Here's the drawing with two shaded views (mm, measured from the low corner). I have some questions. A direction names the side the tool comes from. Coordinates: 2 decimals unless noted, no trailing zeros. Loops run counter-clockwise (first coordinate to the right, second up) from the corner with the lowest first, then second, coordinate; pieces in that order, holes last. Notation, with made-up numbers: (11, -0.75) - (60, -0.75) arc R23 ccw to (60, 16.25) - close; hole circle Ø9 at (56.25, -13). An arc over 180 degrees is marked (long way). Use a Markdown table: item, result.
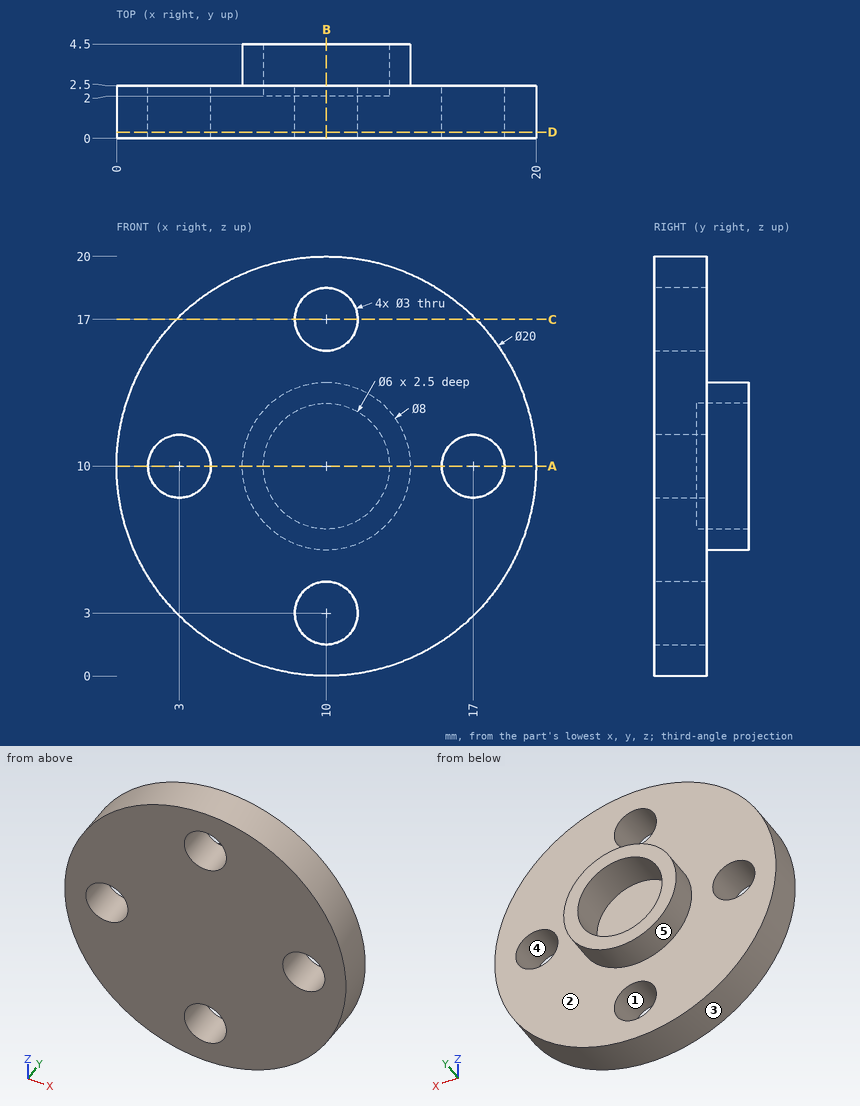
Q1. Will these pins go through, and if not, where does the flat tip stop? P1, Ø2, axis at x = 4, z = 3, coming from the +Y side; P2, Ø3, axis at x = 10, z = 9.5, coming from the +Y side.
Check values:
| item | result |
|---|---|
| P1 | y = 2.5 |
| P2 | y = 2 |
Q2. I want a section at D-D, the plane y = 0.3. Write out the boundary of the cut face in (x, z).
Check values:
| item | result |
|---|---|
| outline | circle Ø20 at (10, 10); hole circle Ø3 at (3, 10); hole circle Ø3 at (10, 3); hole circle Ø3 at (10, 17); hole circle Ø3 at (17, 10) |
Q3. I want a section at B-B, the plane x = 10. Write out the boundary of the cut face in (y, z).
Check values:
| item | result |
|---|---|
| outline | (0, 0) - (2.5, 0) - (2.5, 1.5) - (0, 1.5) - close; (0, 4.5) - (2.5, 4.5) - (2.5, 6) - (4.5, 6) - (4.5, 7) - (2, 7) - (2, 13) - (4.5, 13) - (4.5, 14) - (2.5, 14) - (2.5, 15.5) - (0, 15.5) - close; (0, 18.5) - (2.5, 18.5) - (2.5, 20) - (0, 20) - close |
Q4. I want a section at C-C, the plane z = 17. Write out the boundary of the cut face in (x, y).
Check values:
| item | result |
|---|---|
| outline | (2.86, 0) - (8.5, 0) - (8.5, 2.5) - (2.86, 2.5) - close; (11.5, 0) - (17.14, 0) - (17.14, 2.5) - (11.5, 2.5) - close |
Q5. I want a section at A-A, the plane z = 10. Write out the boundary of the cut face in (x, y).
Check values:
| item | result |
|---|---|
| outline | (0, 0) - (1.5, 0) - (1.5, 2.5) - (0, 2.5) - close; (4.5, 0) - (15.5, 0) - (15.5, 2.5) - (14, 2.5) - (14, 4.5) - (13, 4.5) - (13, 2) - (7, 2) - (7, 4.5) - (6, 4.5) - (6, 2.5) - (4.5, 2.5) - close; (18.5, 0) - (20, 0) - (20, 2.5) - (18.5, 2.5) - close |
Q6. Please list where these lines run through material, in increasing order: L1, parallel to X at y = 3, z = 10; L2, parallel to Z at x = 11, y = 1.3; L3, parallel to Z at x = 10.5, y = 1.7. Write a range as from..to.
Check values:
| item | result |
|---|---|
| L1 | 6..7, 13..14 |
| L2 | 0.05..1.88, 4.12..15.88, 18.12..19.95 |
| L3 | 0.01..1.59, 4.41..15.59, 18.41..19.99 |
Q7. If we mould it in two halves opening along X, with no side actions, what happens to the marked faces 1, 2 and 3? For each: pulls with the +X half, pulls with the -X half, needs draft (parallel to the pull), parting line crosses it, or undercut.
Check values:
| item | result |
|---|---|
| face 1 | undercut |
| face 2 | needs draft |
| face 3 | parting line crosses it |
Q8. Which directions (+Z, -Z, +X, -X, +Y, -Y) give clear straight access to the entire face, cutting with the end or side of a thin tool? Please do the marked faces 4 and 5.
Check values:
| item | result |
|---|---|
| face 4 | +Y, -Y |
| face 5 | +Y |
